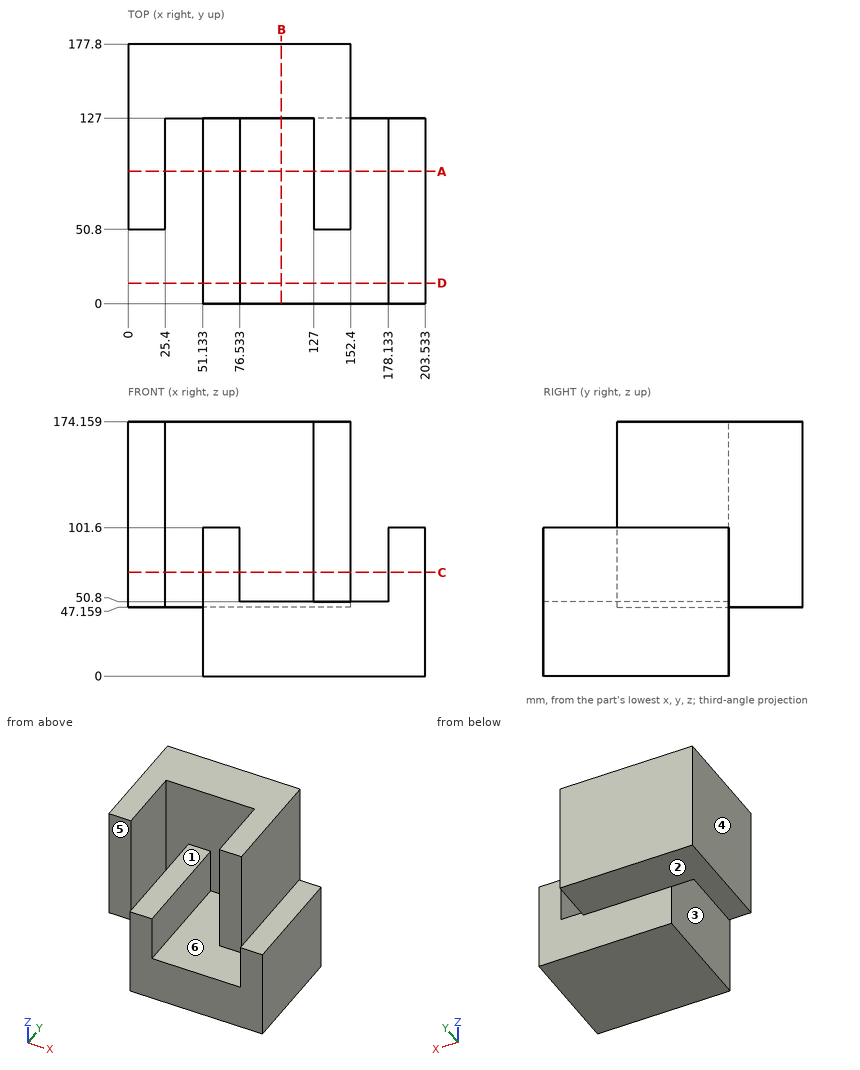
Geometry: see drawing. Coordinates: mm, zero at the bounding-box minimum. A direction names the side the tool comes from. Give positions to 0.01 mm unless a question says otherwise; leave off trailing zeros. Order: outer loops, then holes, each group sorted by start corner. A loop starts at its lowest first (then second) coordinate and runs counter-clockwise, first axis right, second up.
1. Pin query (flat end, axial travel): pin 1 Ø7.5 at (x, y) = (68, 58) entering from +Z; pin 2 Ø12.5 at (x, z) = (139, 112.5) entering from -Y; pin 3 Ø1 at (x, y) = (172.5, 113.5) entering from +Z. Return the tip coordinate at first contact, or that it passes through.
Computed:
pin 1: stops at z = 101.6
pin 2: stops at y = 50.8
pin 3: stops at z = 50.8
2. Cut plane B-B (x = 105). Return loops of the section in (y, z), and give its area (3 significant figures).
Computed:
outline: (0, 0) - (127, 0) - (127, 47.16) - (177.8, 47.16) - (177.8, 174.16) - (127, 174.16) - (127, 50.8) - (0, 50.8) - close
area: 12,900 mm2
3. Draft query along X for the marked faces 4, 5 and 6. Return one class per face: released by +X, released by -X, zero draft, split by the parting line, or undercut.
Computed:
face 4: released by -X
face 5: zero draft
face 6: undercut
4. Set-up query: the marked faces 1, 2 and 3. Return all of +Z, -Z, +X, -X, +Y, -Y with unobstructed straight access to the full face (end or side cutting, diameter ignored); none if empty.
Computed:
face 1: +Z, -Y
face 2: -Z, -X, +Y
face 3: +Z, -Z, -Y
5. Cut plane C-C (z = 71). Return loops of the section in (x, y).
Computed:
outline: (0, 50.8) - (25.4, 50.8) - (25.4, 127) - (51.13, 127) - (51.13, 0) - (76.53, 0) - (76.53, 127) - (127, 127) - (127, 50.8) - (152.4, 50.8) - (152.4, 177.8) - (0, 177.8) - close; (178.13, 0) - (203.53, 0) - (203.53, 127) - (178.13, 127) - close
6. Line query: probe 1 along X at (y, z) = (58.5, 87); probe 2 along X at (y, z) = (100.5, 134.5); probe 3 along Y at (x, z) = (133.5, 157). Output: solid intervals per line, ascending.
Computed:
probe 1: x = 0 to 25.4, 51.13 to 76.53, 127 to 152.4, 178.13 to 203.53
probe 2: x = 0 to 25.4, 127 to 152.4
probe 3: y = 50.8 to 177.8
7. Cut plane A-A (y = 90.5). Return loops of the section in (x, z).
Computed:
outline: (0, 47.16) - (25.4, 47.16) - (25.4, 174.16) - (0, 174.16) - close; (51.13, 0) - (203.53, 0) - (203.53, 101.6) - (178.13, 101.6) - (178.13, 50.8) - (152.4, 50.8) - (152.4, 174.16) - (127, 174.16) - (127, 50.8) - (76.53, 50.8) - (76.53, 101.6) - (51.13, 101.6) - close
8. Cut plane D-D (y = 14). Return loops of the section in (x, z).
Computed:
outline: (51.13, 0) - (203.53, 0) - (203.53, 101.6) - (178.13, 101.6) - (178.13, 50.8) - (76.53, 50.8) - (76.53, 101.6) - (51.13, 101.6) - close
